The listing builds one solid part. Answer for the finished solid, in the listing's coordinates (mm). Coordinates: 2 decimals unless noted, no trailing zeros. Write each loop counter-clockwise with the first axis right and the second up, starting at its lowest first coordinate (ties: lowest second). Pieces come first, ordered by that corner, then holes. Notation, with made-up numbers: M 49,-2.5 L 76,-2.5 A24 cw 76,27.5 Z; hole C 69,89 d7. An arc over 180 degrees is marked long. Answer as CSV lines item,"result". Start each with the question number.
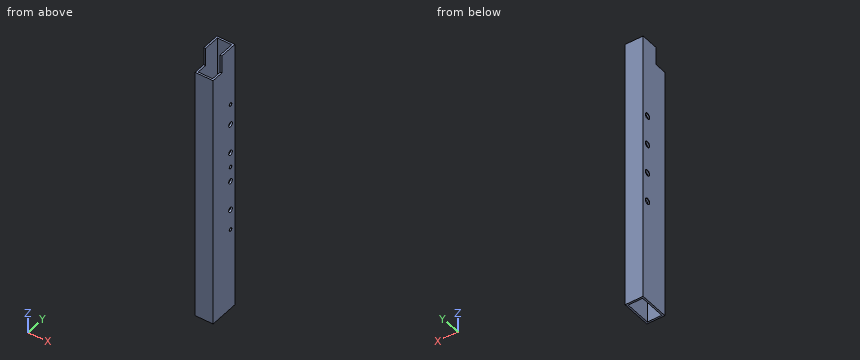
```python
from build123d import *

# Parameters (mm, degrees)
SKETCH_1_W                   = 30
SKETCH_1_H                   = 50
SKETCH_1_W_2                 = 24
SKETCH_1_H_2                 = 44
EXTRUDE_1_DEPTH              = 458
SKETCH_2_W                   = 30
SKETCH_2_H                   = 20
CUT_EXTRUDE_1_DEPTH          = 462.696870251
HOLE_WIZARD_M61_D            = 5
HOLE_WIZARD_M61_DEPTH        = 17
HOLE_WIZARD_M61_CSINK_D      = 6.05
HOLE_WIZARD_M61_CSINK_ANGLE  = 120
HOLE_WIZARD_M61_TIP          = 1.502151548
HOLE_WIZARD_M101_D           = 8.5
HOLE_WIZARD_M101_DEPTH       = 47.5
HOLE_WIZARD_M101_CSINK_D     = 10.05
HOLE_WIZARD_M101_CSINK_ANGLE = 120
HOLE_WIZARD_M101_TIP         = 2.553657631


with BuildPart() as part:
    # Эскиз1 → Вытянуть-Тонкостенный1 (new body)
    with BuildSketch(Plane.XY):
        with Locations((15, 25)):
            Rectangle(SKETCH_1_W, SKETCH_1_H)
        with Locations((15, 25)):
            Rectangle(SKETCH_1_W_2, SKETCH_1_H_2, mode=Mode.SUBTRACT)
    extrude(amount=EXTRUDE_1_DEPTH)

    # Эскиз2 → Вырез-Вытянуть1 (cut, through all)
    with BuildSketch(Plane(origin=(30, 0, 0), x_dir=(0, 0, -1), z_dir=(1, 0, 0))):
        with Locations((-443, 10)):
            Rectangle(SKETCH_2_W, SKETCH_2_H)
    extrude(amount=-CUT_EXTRUDE_1_DEPTH, mode=Mode.SUBTRACT)

    # Отверстие обработанное метчиком M61
    with Locations(Plane(origin=(30, 0, 0), x_dir=(0, 0, -1), z_dir=(1, 0, 0))):
        with Locations((-249, 40), (-359, 40), (-139, 40)):
            CounterSinkHole(HOLE_WIZARD_M61_D / 2, HOLE_WIZARD_M61_CSINK_D / 2, depth=HOLE_WIZARD_M61_DEPTH, counter_sink_angle=HOLE_WIZARD_M61_CSINK_ANGLE)
            with Locations((0, 0, -(HOLE_WIZARD_M61_DEPTH + HOLE_WIZARD_M61_TIP / 2))):  # 118° drill point
                Cone(0, HOLE_WIZARD_M61_D / 2, HOLE_WIZARD_M61_TIP, mode=Mode.SUBTRACT)

    # Отверстие обработанное метчиком M101
    with Locations(Plane.ZY):
        with Locations((224, 40), (174, 40), (324, 40), (274, 40)):
            CounterSinkHole(HOLE_WIZARD_M101_D / 2, HOLE_WIZARD_M101_CSINK_D / 2, depth=HOLE_WIZARD_M101_DEPTH, counter_sink_angle=HOLE_WIZARD_M101_CSINK_ANGLE)
            with Locations((0, 0, -(HOLE_WIZARD_M101_DEPTH + HOLE_WIZARD_M101_TIP / 2))):  # 118° drill point
                Cone(0, HOLE_WIZARD_M101_D / 2, HOLE_WIZARD_M101_TIP, mode=Mode.SUBTRACT)


solid = part.part
```
1) The part is cut by section B-B (y = 28.5). Determine the outline of the cut face in (x, z).
2) Find the intervals of material crossed by line 1 (X direction, y = 20.5, z = 29.5); line 2 (Y direction, x = 26, z = 55.5); line 3 (Z direction, x = 1.9, y = 40), in increasing order. Write a range as from..to.
3) Each of these flat-tipped pins is pushed along its axis until it touches: P1, Ø7, axis at y = 40, z = 174, coming from the +X side; P2, Ø10, axis at y = 40, z = 224, coming from the -X side; P3, Ø16, axis at x = 22.5, y = 12.5, coming from the +Z side; P4, Ø1.5, axis at x = 28.5, z = 449, coming from the -Y side. Where does it stop, or does it pass through?
4) The part is cut by section A-A (x = 9). Determine the outline of the cut face in (y, z), then the cut area to 3 significant figures.
5) The part is cut by section C-C (z = 274). Determine the outline of the cut face in (x, y) (3 decimals), then the cut area to 3 significant figures.
Completed:
1,outline,"M 0,0 L 3,0 L 3,458 L 0,458 Z; M 27,0 L 30,0 L 30,458 L 27,458 Z"
2,line 1,"0..3, 27..30"
2,line 2,"0..3, 47..50"
2,line 3,"0..169.75, 178.25..219.75, 228.25..269.75, 278.25..319.75, 328.25..458"
3,P1,"through"
3,P2,"x = 0.01"
3,P3,"z = 428"
3,P4,"y = 20"
4,outline,"M 0,0 L 3,0 L 3,428 L 0,428 Z; M 47,0 L 50,0 L 50,458 L 47,458 Z"
4,area,"2,660 mm²"
5,outline,"M 0,0 L 30,0 L 30,35.75 L 27,35.75 L 27,3 L 3,3 L 3,35.75 L 0.447,35.75 L 0,34.975 Z; M 0,45.025 L 0.447,44.25 L 3,44.25 L 3,47 L 27,47 L 27,44.25 L 30,44.25 L 30,50 L 0,50 Z"
5,area,"393 mm²"
